```python
from build123d import *

# Parameters (mm, degrees)
BOSS_EXTRUDE1_DEPTH = 10
BOSS_EXTRUDE2_DEPTH = 15


with BuildPart() as part:
    # Sketch1 → Boss-Extrude1 (new body)
    with BuildSketch(Plane.XY):
        with BuildLine():
            Line((-30, 0), (0, 0))
            Line((0, 0), (0, 20))
            Line((0, 20), (-10, 20))
            ThreePointArc((-10, 20), (-24.142135624, 14.142135624), (-30, 0))
        make_face()
    extrude(amount=BOSS_EXTRUDE1_DEPTH)

    # Sketch2 → Boss-Extrude2 (add)
    with BuildSketch(Plane.XY.offset(10)):
        with BuildLine():
            Line((0, 0), (-30, 25))
            ThreePointArc((-30, 25), (-10.47437581, 17.930749028), (0, 0))
        make_face()
    extrude(amount=BOSS_EXTRUDE2_DEPTH)


solid = part.part
```
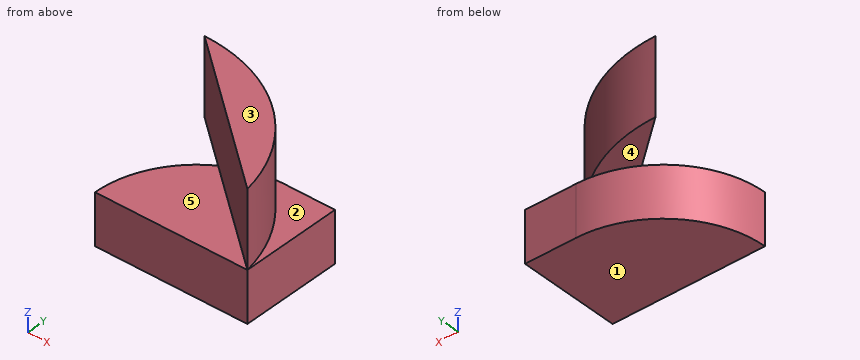
The listing builds one solid part. Answer for the finished solid, in the listing's coordinates (mm). Face numbers are marked on the shaded views. A direction names the side the tool comes from. Round coordinates to 2 decimals unless told otherwise and drop trailing zeros. Loops run counter-clockwise (first coordinate to the right, second up) from the corner with the lowest first, then second, coordinate; pieces in that order, holes last.
1) Consider line 1 (Y direction, x = -6, z = 8); line 2 (Z direction, x = -18, y = 3); line 3 (Y direction, x = -3.5, z = 13.5). Determine where each line is inside the solid, lowest interval first.
Outcome:
line 1: y = 0 to 20
line 2: z = 0 to 10
line 3: y = 2.92 to 9.6
2) A cutting plane is placed at A-A on x = -25.5. Determine the outline of the cut face in (y, z), plus the area to 3 significant figures.
Outcome:
outline: (0, 0) - (12.64, 0) - (12.64, 10) - (0, 10) - close; (21.25, 10) - (24.67, 10) - (24.67, 25) - (21.25, 25) - close
area: 178 mm2
3) A cutting plane is placed at B-B on z = 15.5. Determine the outline of the cut face in (x, y).
Outcome:
outline: (-30, 25) - (0, 0) arc R30.5 ccw to start
4) A cutting plane is placed at C-C on y = 2.25. Determine the outline of the cut face in (x, z), plus the area to 3 significant figures.
Outcome:
outline: (-29.87, 0) - (0, 0) - (0, 10) - (-0.5, 10) - (-0.5, 25) - (-2.7, 25) - (-2.7, 10) - (-29.87, 10) - close
area: 332 mm2
5) A cutting plane is placed at D-D on x = -15.5. Determine the outline of the cut face in (y, z).
Outcome:
outline: (0, 0) - (19.23, 0) - (19.23, 10) - (21.33, 10) - (21.33, 25) - (12.92, 25) - (12.92, 10) - (0, 10) - close
6) Given P1, Ø5, axis at x = -5.5, y = 18, coming from the +Z side; P2, Ø5, axis at x = -9, z = 10, coming from the +Y side; P3, Ø8, axis at x = -11, z = 16, coming from the -Y side, each flat-ended and moving along its own axis, determine where each tip first touches the part or whether it passes through.
Outcome:
P1: stops at z = 10
P2: stops at y = 20
P3: stops at y = 5.83
7) For the marked faces 1, 2, 3, 4 and 5, determine the directions among +Z, -Z, +X, -X, +Y, -Y from which every point of the face is accessible in a straight line to the end or side of a thin tool.
Outcome:
face 1: -Z, +X, -X, +Y, -Y
face 2: +Z, +X, +Y
face 3: +Z, +X, -X, +Y, -Y
face 4: -Z, -X, +Y
face 5: +Z, -X, -Y
